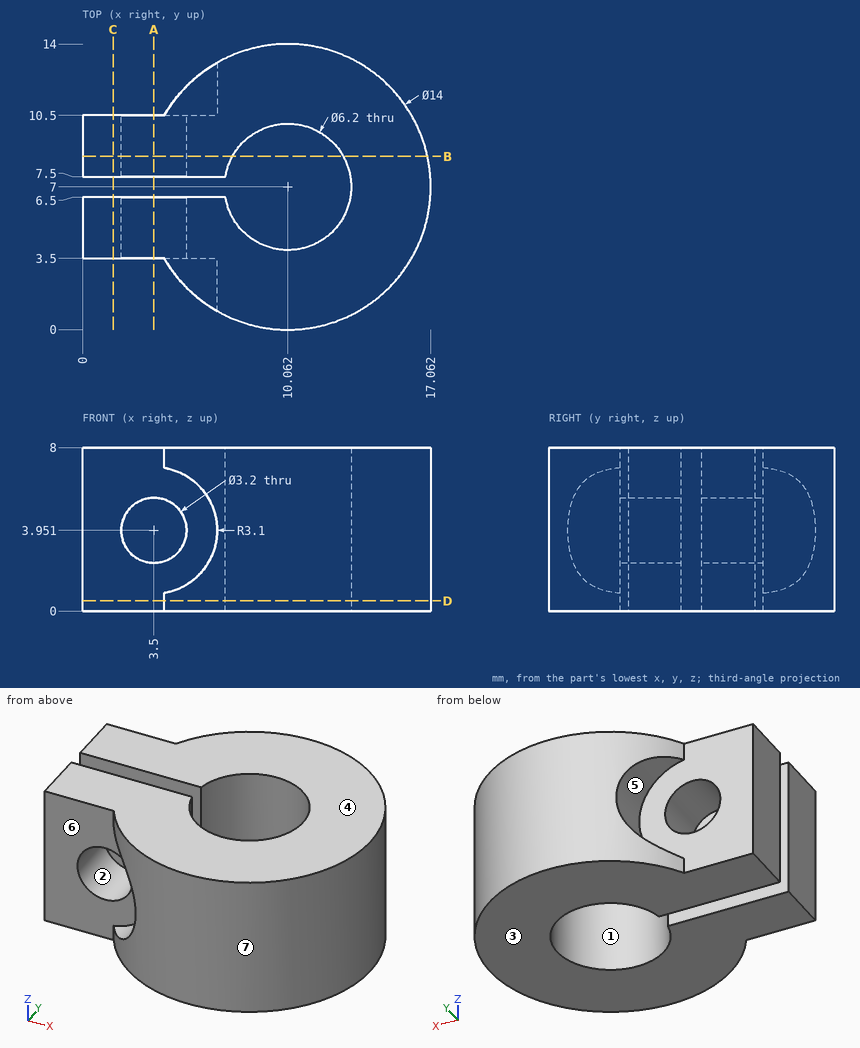
Geometry: see drawing. Coordinates: mm, zero at the bounding-box minimum. A direction names the side the tool comes from. Coordinates: 2 decimals unless noted, no trailing zeros. Order: outer loops, then holes, each group sorted by start corner. A loop starts at its lowest first (then second) coordinate and runs counter-clockwise, first axis right, second up. Notation, with made-up numbers: M 64,86 L 103,86 A12 cw 103,103 Z; hole C 75.25,-33 d8. An arc over 180 degrees is marked long. Answer in a Markdown table with one row per item. Add a question column.
Q1. Line query: L1, parallel to Z at x = 3.5, y = 9.7; L2, parallel to Y at x = 1.5, z = 6.5; L3, parallel to Y at x = 7.25, z = 3.25 (1 decimal). Output: solid intervals per line, ascending.
Q2. Section query B-B on y = 8.5. Count the separate pieces of the cut face and the enclosed holes in it.
Q3. Section query C-C on x = 1.5. Return the cut outline in (y, z), and give its area (3 significant figures).
Q4. Section query A-A on x = 3.5. Return the cut outline in (y, z), and give its area (3 significant figures).
Q5. Reachability of the marked faces 5, 6 and 7 from +Z, -Z, +X, -X, +Y, -Y: full face, straight path, thin tool, end or side. Return the list, or none.
Q6. Mould query, pull axis Z, two halves, no side actions, for the marked faces 1, 2, 3 and 4. Classes: released by +Z, released by -Z, zero draft, split by the parting line, or undercut.
Q7. Contact query for flat-ended pins moving along their axis: P1, Ø4, axis at y = 9.5, z = 4, coming from the +X side; P2, Ø2, axis at x = 3.5, z = 3, coming from the +Y side; P3, Ø3.5, axis at x = 3, z = 6, coming from the -Y side (1 decimal). Output: stop coordinate, or through.
Q8. Section query D-D on z = 0.5. Return the cut outline in (x, y).
Completed:
| question | item | result |
|---|---|---|
| 1 | L1 | z = 0 to 2.35, 5.55 to 8 |
| 1 | L2 | y = 3.5 to 6.5, 7.5 to 10.5 |
| 1 | L3 | y = 0.6 to 5.7, 8.3 to 13.4 |
| 2 | separate pieces | 2 |
| 2 | enclosed holes | 1 |
| 3 | outline | M 3.5,0 L 6.5,0 L 6.5,8 L 3.5,8 Z; M 7.5,0 L 10.5,0 L 10.5,8 L 7.5,8 Z |
| 3 | area | 48.0 mm2 |
| 4 | outline | M 3.5,0 L 6.5,0 L 6.5,2.35 L 3.5,2.35 Z; M 3.5,5.55 L 6.5,5.55 L 6.5,8 L 3.5,8 Z; M 7.5,0 L 10.5,0 L 10.5,2.35 L 7.5,2.35 Z; M 7.5,5.55 L 10.5,5.55 L 10.5,8 L 7.5,8 Z |
| 4 | area | 28.8 mm2 |
| 5 | face 5 | -X, +Y |
| 5 | face 6 | -X, -Y |
| 5 | face 7 | +Z, -Z |
| 6 | face 1 | zero draft |
| 6 | face 2 | undercut |
| 6 | face 3 | released by -Z |
| 6 | face 4 | released by +Z |
| 7 | P1 | stops at x = 17.04 |
| 7 | P2 | stops at y = 10.5 |
| 7 | P3 | stops at y = 2.7 |
| 8 | outline | M 0,3.5 L 4,3.5 A7 ccw long 4,10.5 L 0,10.5 L 0,7.5 L 7,7.5 A3.1 cw long 7,6.5 L 0,6.5 Z |
